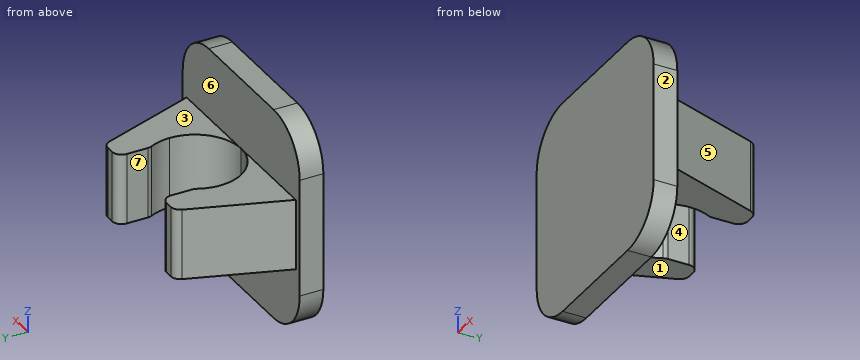
from build123d import *

# Parameters (mm, degrees)
SKETCH1_W           = 9
SKETCH1_H           = 9
BOSS_EXTRUDE1_DEPTH = 1
BOSS_EXTRUDE2_DEPTH = 3
FILLET1_R           = 0.4
FILLET2_R           = 2


with BuildPart() as part:
    # Sketch1 → Boss-Extrude1 (new body)
    with BuildSketch(Plane(origin=(0, 0, 0), x_dir=(1, 0, 0), z_dir=(0, 1, 0))):
        Rectangle(SKETCH1_W, SKETCH1_H)
    extrude(amount=BOSS_EXTRUDE1_DEPTH)

    # Sketch2 → Boss-Extrude2 (add)
    with BuildSketch(Plane.XY.offset(1.5)):
        with BuildLine():
            ThreePointArc((0, 1), (-1.683038158, 1.965173844), (-1.7, 3.905248659))
            Line((-1.7, 3.905248659), (-1.7, 5.3))
            Line((-1.7, 5.3), (-2.7, 5.3))
            Line((-2.7, 5.3), (-4.2, 1))
            Line((-4.2, 1), (0, 1))
        make_face()
        with BuildLine():
            Line((1.7, 5.3), (1.7, 3.905248659))
            ThreePointArc((1.7, 3.905248659), (1.886464948, 3.443710441), (1.95, 2.95))
            ThreePointArc((1.95, 2.95), (1.378858223, 1.571141777), (0, 1))
            Line((0, 1), (4.2, 1))
            Line((4.2, 1), (2.7, 5.3))
            Line((2.7, 5.3), (1.7, 5.3))
        make_face()
    extrude(amount=-BOSS_EXTRUDE2_DEPTH)

    # Fillet1
    fillet1_edges = [part.edges().sort_by_distance(p)[0] for p in [
        (-1.7, 3.905248659, 0),
        (-2.7, 5.3, 0),
        (-1.7, 5.3, 0),
        (1.7, 3.905248659, 0),
        (1.7, 5.3, 0),
        (2.7, 5.3, 0),
    ]]
    fillet(fillet1_edges, radius=FILLET1_R)

    # Fillet2
    fillet2_edges = [part.edges().sort_by_distance(p)[0] for p in [
        (4.5, 0.5, 4.5),
        (-4.5, 0.5, 4.5),
        (-4.5, 0.5, -4.5),
        (4.5, 0.5, -4.5),
    ]]
    fillet(fillet2_edges, radius=FILLET2_R)


solid = part.part
Could you check a few things on this model? Use its own coordinates, in mm. Face numbers are marked on the shaded views. A direction names the side the tool comes from. Round coordinates to 2 decimals unless told otherwise and drop trailing zeros. Write each loop counter-clockwise with the first axis right and the second up, starting at its lowest first coordinate (ties: lowest second). Pieces come first, ordered by that corner, then holes. Notation, with made-up numbers: (3.5, 78.5) -> (58.5, 78.5) arc R24 cw to (58.5, 89.5) -> close; hole circle Ø8 at (-7.75, -30.5). An arc over 180 degrees is marked (long way). Use a Markdown table: item, result.
1. Please list where these lines run through material, in increasing order: probe 1 along Z at (x, y) = (2.75, 4.4); probe 2 along Y at (x, z) = (-2.5, -3.75); probe 3 along X at (y, z) = (1.25, 1).
Answer key:
| item | result |
|---|---|
| probe 1 | z = -1.5 to 1.5 |
| probe 2 | y = 0 to 1 |
| probe 3 | x = -4.11 to -0.96, 0.96 to 4.11 |
2. For pin 1 Ø1.5 at (x, y) = (1.5, 3.5) entering from +Z; pin 2 Ø0.7 at (y, z) = (4.5, -0.5) entering from -X; pin 3 Ø2 at (x, z) = (-0.5, 0) entering from +Y, each with a flat end and sliding along its axis, tell me the tip position at first contact or that it passes through.
Answer key:
| item | result |
|---|---|
| pin 1 | stops at z = 1.5 |
| pin 2 | stops at x = -3.1 |
| pin 3 | stops at y = 1.7 |
3. If we section it at A-A (y = 1.8): List the corners of the cut face in (x, z) for me.
Answer key:
| item | result |
|---|---|
| outline | (-3.92, -1.5) -> (-1.57, -1.5) -> (-1.57, 1.5) -> (-3.92, 1.5) -> close; (1.57, -1.5) -> (3.92, -1.5) -> (3.92, 1.5) -> (1.57, 1.5) -> close |
4. We'd pull the mould along X, two halves only. Please class the marked faces 5, 6 and 7: +X half, -X half, draft (parallel to the pull), parting line (faces both ways), or undercut.
Answer key:
| item | result |
|---|---|
| face 5 | +X half |
| face 6 | draft |
| face 7 | undercut |
5. If we section it at D-D (x = -3.5): List the corners of the cut face in (y, z) for me.
Answer key:
| item | result |
|---|---|
| outline | (0, -4.23) -> (1, -4.23) -> (1, -1.5) -> (3.01, -1.5) -> (3.01, 1.5) -> (1, 1.5) -> (1, 4.23) -> (0, 4.23) -> close |
6. If we section it at C-C (y = 0.65): List the corners of the cut face in (x, z) for me.
Answer key:
| item | result |
|---|---|
| outline | (-4.5, -2.5) arc R2 ccw to (-2.5, -4.5) -> (2.5, -4.5) arc R2 ccw to (4.5, -2.5) -> (4.5, 2.5) arc R2 ccw to (2.5, 4.5) -> (-2.5, 4.5) arc R2 ccw to (-4.5, 2.5) -> close |
7. Which directions (+Z, -Z, +X, -X, +Y, -Y) give clear straight access to the entire face, cutting with the end or side of a thin tool? Please do the marked faces 1, 2, 3 and 4.
Answer key:
| item | result |
|---|---|
| face 1 | -Z, +X, -X, +Y |
| face 2 | +Z, -Z, +X, +Y, -Y |
| face 3 | +Z, +X, -X, +Y |
| face 4 | +Z, -Z, +Y |
8. If we section it at B-B (z = -0.75): List the corners of the cut face in (x, y) for me.
Answer key:
| item | result |
|---|---|
| outline | (-4.5, 0) -> (4.5, 0) -> (4.5, 1) -> (4.2, 1) -> (2.79, 5.03) arc R0.4 ccw to (2.42, 5.3) -> (2.1, 5.3) arc R0.4 ccw to (1.7, 4.9) -> (1.7, 4) arc R0.4 ccw to (1.74, 3.83) arc R1.95 cw (long way) to (-1.74, 3.83) arc R0.4 ccw to (-1.7, 4) -> (-1.7, 4.9) arc R0.4 ccw to (-2.1, 5.3) -> (-2.42, 5.3) arc R0.4 ccw to (-2.79, 5.03) -> (-4.2, 1) -> (-4.5, 1) -> close |
